Verification items for the finished model (mm, model axes). A direction names the side the tool comes from. Coordinates: 2 decimals unless noted, no trailing zeros. Loops run counter-clockwise (first coordinate to the right, second up) from the corner with the lowest first, then second, coordinate; pieces in that order, holes last. Notation, with made-up numbers: (85, 75.25) -> (111, 75.25) arc R22 cw to (111, 90.25) -> close; hole circle Ø7 at (33.5, 59). An arc over 180 degrees is marked (long way). Write item = value, one per line.
```python
from build123d import *

# Parameters (mm, degrees)
BOSS_EXTRUDE1_START     = 3.25
BOSS_EXTRUDE1_OUTLINE_W = 176
BOSS_EXTRUDE1_OUTLINE_H = 126
BOSS_EXTRUDE1_DEPTH     = 6
BOSS_EXTRUDE2_DEPTH     = 3.3
BOSS_EXTRUDE4_DEPTH     = 1
SKETCH7_W               = 12.05
SKETCH7_H               = 9
CUT_EXTRUDE1_DEPTH      = 6
BOSS_EXTRUDE5_DEPTH     = 3.3
BOSS_EXTRUDE7_DEPTH     = 1
BOSS_EXTRUDE8_START     = 2.6
BOSS_EXTRUDE8_DEPTH     = 2.6
BOSS_EXTRUDE9_START     = 0.7
BOSS_EXTRUDE9_DEPTH     = 0.7
BOSS_EXTRUDE10_START    = 1
BOSS_EXTRUDE10_DEPTH    = 1
SKETCH14_W              = 12.7
SKETCH14_H              = 3.5
SKETCH14_W_2            = 3.5
SKETCH14_H_2            = 25.4
CUT_EXTRUDE2_DEPTH      = 6.5116
CUT_EXTRUDE3_REACH      = 194.673
SKETCH15_R              = 4
CUT_EXTRUDE4_DEPTH      = 4.3
FILLET1_R               = 3
CUT_EXTRUDE5_START      = -4.8616
CUT_EXTRUDE5_DEPTH      = 4.8616
SKETCH19_W              = 176.2
SKETCH19_H              = 126.4
CUT_EXTRUDE6_DEPTH      = 3
SKETCH16_R              = 4
SKETCH16_R_2            = 2.1
BOSS_EXTRUDE11_DEPTH    = 4.25
SKETCH20_W              = 129.139207087
SKETCH20_H              = 3
SKETCH20_W_2            = 9.439207087
SKETCH20_W_3            = 158.5
BOSS_EXTRUDE12_DEPTH    = 4.25


# Read off the part's stored shape, not the designer's step: Boss-Extrude1, Cut-Extrude5
with BuildPart() as part:
    # Boss-Extrude1 outline → Boss-Extrude1 (new body)
    with BuildSketch(Plane.XY.offset(BOSS_EXTRUDE1_START)):
        with Locations((-88, 0)):
            Rectangle(BOSS_EXTRUDE1_OUTLINE_W, BOSS_EXTRUDE1_OUTLINE_H)
    extrude(amount=BOSS_EXTRUDE1_DEPTH)

    # Sketch3 → Boss-Extrude2 (add)
    with BuildSketch(Plane.ZY.offset(176)):
        with BuildLine():
            Line((9.25, -63), (9.25, 63))
            Line((9.25, 63), (-1.6116, 63))
            Line((-1.6116, 63), (-1.6116, 12.5))
            Line((-1.6116, 12.5), (0.4, 12.5))
            ThreePointArc((0.4, 12.5), (3.228427125, 11.328427125), (4.4, 8.5))
            Line((4.4, 8.5), (4.4, -8.5))
            ThreePointArc((4.4, -8.5), (3.228427125, -11.328427125), (0.4, -12.5))
            Line((0.4, -12.5), (-1.6116, -12.5))
            Line((-1.6116, -12.5), (-1.6116, -63))
            Line((-1.6116, -63), (9.25, -63))
        make_face()
    extrude(amount=BOSS_EXTRUDE2_DEPTH)

    # Sketch6 → Boss-Extrude4 (add)
    with BuildSketch(Plane.ZY.offset(179.3)):
        with BuildLine():
            Line((9.25, -63), (9.25, 63))
            Line((9.25, 63), (-1.6116, 63))
            Line((-1.6116, 63), (-1.6116, 11.25))
            Line((-1.6116, 11.25), (0.4, 11.25))
            ThreePointArc((0.4, 11.25), (2.415254326, 10.415254326), (3.25, 8.4))
            Line((3.25, 8.4), (3.25, -8.4))
            ThreePointArc((3.25, -8.4), (2.415254326, -10.415254326), (0.4, -11.25))
            Line((0.4, -11.25), (-1.6116, -11.25))
            Line((-1.6116, -11.25), (-1.6116, -63))
            Line((-1.6116, -63), (9.25, -63))
        make_face()
    extrude(amount=BOSS_EXTRUDE4_DEPTH)

    # Sketch7 → Cut-Extrude1 (cut)
    with BuildSketch(Plane(origin=(0, 0, 3.25), x_dir=(-1, 0, 0), z_dir=(0, 0, -1))):
        with Locations((138.325, -13.3)):
            Rectangle(SKETCH7_W, SKETCH7_H)
    extrude(amount=-CUT_EXTRUDE1_DEPTH, mode=Mode.SUBTRACT)

    # Sketch8 → Boss-Extrude5 (add)
    with BuildSketch(Plane.XZ.offset(63)):
        with BuildLine():
            Line((0, 9.25), (-180.3, 9.25))
            Line((-180.3, 9.25), (-180.3, -1.6116))
            Line((-180.3, -1.6116), (-11.957378406, -1.6116))
            ThreePointArc((-11.957378406, -1.6116), (-11.96744863, 2.394191566), (-8.5, 4.4))
            Line((-8.5, 4.4), (0, 4.4))
            Line((0, 4.4), (0, 9.25))
        make_face()
    extrude(amount=BOSS_EXTRUDE5_DEPTH)

    # Sketch10 → Boss-Extrude7 (add)
    with BuildSketch(Plane.XZ.offset(66.3)):
        with BuildLine():
            Line((0, 9.25), (-180.3, 9.25))
            Line((-180.3, 9.25), (-180.3, -1.6116))
            Line((-180.3, -1.6116), (-11.25, -1.6116))
            Line((-11.25, -1.6116), (-11.25, 0.4))
            ThreePointArc((-11.25, 0.4), (-10.415254326, 2.415254326), (-8.4, 3.25))
            Line((-8.4, 3.25), (0, 3.25))
            Line((0, 3.25), (0, 9.25))
        make_face()
    extrude(amount=BOSS_EXTRUDE7_DEPTH)

    # Sketch11 → Boss-Extrude8 (add)
    with BuildSketch(Plane(origin=(0, 63, 0), x_dir=(1, 0, 0), z_dir=(0, 1, 0)).offset(BOSS_EXTRUDE8_START)):
        with BuildLine():
            Line((-180.3, -9.25), (0, -9.25))
            Line((0, -9.25), (0, -4.4))
            Line((0, -4.4), (-8.5, -4.4))
            ThreePointArc((-8.5, -4.4), (-11.96744863, -2.394191566), (-11.957378406, 1.6116))
            Line((-11.957378406, 1.6116), (-180.3, 1.6116))
            Line((-180.3, 1.6116), (-180.3, -9.25))
        make_face()
    extrude(amount=-BOSS_EXTRUDE8_DEPTH)

    # Sketch12 → Boss-Extrude9 (add)
    with BuildSketch(Plane(origin=(0, 65.6, 0), x_dir=(1, 0, 0), z_dir=(0, 1, 0)).offset(BOSS_EXTRUDE9_START)):
        with BuildLine():
            Line((-180.3, -9.25), (0, -9.25))
            Line((0, -9.25), (0, -4.4))
            Line((0, -4.4), (-8.5, -4.4))
            ThreePointArc((-8.5, -4.4), (-11.96744863, -2.394191566), (-11.957378406, 1.6116))
            Line((-11.957378406, 1.6116), (-180.3, 1.6116))
            Line((-180.3, 1.6116), (-180.3, -9.25))
        make_face()
    extrude(amount=-BOSS_EXTRUDE9_DEPTH)

    # Sketch13 → Boss-Extrude10 (add)
    with BuildSketch(Plane(origin=(0, 66.3, 0), x_dir=(1, 0, 0), z_dir=(0, 1, 0)).offset(BOSS_EXTRUDE10_START)):
        with BuildLine():
            Line((-180.3, -9.25), (0, -9.25))
            Line((0, -9.25), (0, -3.25))
            Line((0, -3.25), (-8.4, -3.25))
            ThreePointArc((-8.4, -3.25), (-10.415254326, -2.415254326), (-11.25, -0.4))
            Line((-11.25, -0.4), (-11.25, 1.6116))
            Line((-11.25, 1.6116), (-180.3, 1.6116))
            Line((-180.3, 1.6116), (-180.3, -9.25))
        make_face()
    extrude(amount=-BOSS_EXTRUDE10_DEPTH)

    # Sketch14 → Cut-Extrude2 (cut)
    with BuildSketch(Plane(origin=(0, 0, -1.6116), x_dir=(-1, 0, 0), z_dir=(0, 0, -1))):
        with Locations((6.35, 64.75)):
            Rectangle(SKETCH14_W, SKETCH14_H)
        with Locations((177.75, 0)):
            Rectangle(SKETCH14_W_2, SKETCH14_H_2)
        with Locations((6.35, -64.75)):
            Rectangle(SKETCH14_W, SKETCH14_H)
    extrude(amount=-CUT_EXTRUDE2_DEPTH, mode=Mode.SUBTRACT)

    # Sketch15 → Cut-Extrude3 (cut, up to next)
    with BuildSketch(Plane.ZY.offset(180.3), mode=Mode.PRIVATE) as cut_extrude3_sk1:
        with Locations((-3.6116, -37.125)):
            Circle(SKETCH15_R)
    cut_extrude3_tool1 = extrude(cut_extrude3_sk1.sketch, amount=-CUT_EXTRUDE3_REACH, mode=Mode.PRIVATE) & part.part
    add(cut_extrude3_tool1.solids().sort_by_distance((-180.3, -37.125, -3.6116))[0], mode=Mode.SUBTRACT)

    # Sketch17 → Cut-Extrude4 (cut)
    with BuildSketch(Plane(origin=(0, 67.3, 0), x_dir=(1, 0, 0), z_dir=(0, 1, 0))):
        with BuildLine():
            Line((-28.4716, -5.0716), (-34.7284, -5.0716))
            ThreePointArc((-34.7284, -5.0716), (-38.07, -1.73), (-34.7284, 1.6116))
            Line((-34.7284, 1.6116), (-28.4716, 1.6116))
            ThreePointArc((-28.4716, 1.6116), (-25.13, -1.73), (-28.4716, -5.0716))
        make_face()
    extrude(amount=-CUT_EXTRUDE4_DEPTH, mode=Mode.SUBTRACT)

    # Fillet1
    fillet1_edges = [part.edges().sort_by_distance(p)[0] for p in [
        (-34.7284, 65.15, -1.6116),
    ]]
    fillet(fillet1_edges, radius=FILLET1_R)
    fillet1_2_edges = [part.edges().sort_by_distance(p)[0] for p in [
        (-28.4716, 65.15, -1.6116),
    ]]
    fillet(fillet1_2_edges, radius=FILLET1_R)

    # Cut-Extrude5 outline → Cut-Extrude5 (cut)
    with BuildSketch(Plane(origin=(0, 0, -1.6116), x_dir=(-1, 0, 0), z_dir=(0, 0, -1)).offset(CUT_EXTRUDE5_START)):
        Polygon((176, 63), (176, -63), (0, -63), (0, -63.2), (176.2, -63.2), (176.2, 63.2), (0, 63.2), (0, 63), align=None)
    extrude(amount=CUT_EXTRUDE5_DEPTH, mode=Mode.SUBTRACT)

    # Sketch19 → Cut-Extrude6 (cut)
    with BuildSketch(Plane(origin=(0, 0, 3.25), x_dir=(-1, 0, 0), z_dir=(0, 0, -1))):
        with Locations((88.1, 0)):
            Rectangle(SKETCH19_W, SKETCH19_H)
    extrude(amount=-CUT_EXTRUDE6_DEPTH, mode=Mode.SUBTRACT)

    # Sketch16 → Boss-Extrude11 (add)
    # profile 1 of 3: a face of its own
    with BuildSketch(Plane(origin=(0, 0, 6.25), x_dir=(-1, 0, 0), z_dir=(0, 0, -1))):
        with Locations(Location((156.5, 38, 0), (0, 0, 270))):
            Circle(SKETCH16_R)
        with Locations((156.5, 38)):
            Circle(SKETCH16_R_2, mode=Mode.SUBTRACT)
    # profile 2 of 3: a face of its own
    with BuildSketch(Plane(origin=(0, 0, 6.25), x_dir=(-1, 0, 0), z_dir=(0, 0, -1))):
        with Locations(Location((23.5, 38, 0), (0, 0, 270))):
            Circle(SKETCH16_R)
        with Locations((23.5, 38)):
            Circle(SKETCH16_R_2, mode=Mode.SUBTRACT)
    # profile 3 of 3: a face of its own
    with BuildSketch(Plane(origin=(0, 0, 6.25), x_dir=(-1, 0, 0), z_dir=(0, 0, -1))):
        with Locations(Location((123.5, -32, 0), (0, 0, 270))):
            Circle(SKETCH16_R)
        with Locations((123.5, -32)):
            Circle(SKETCH16_R_2, mode=Mode.SUBTRACT)
    extrude(amount=BOSS_EXTRUDE11_DEPTH)

    # Sketch20 → Boss-Extrude12 (add)
    with BuildSketch(Plane(origin=(0, 0, 6.25), x_dir=(-1, 0, 0), z_dir=(0, 0, -1))):
        with Locations((108.630396457, 61.7)):
            Rectangle(SKETCH20_W, SKETCH20_H)
        with Locations((17.419603544, 61.7)):
            Rectangle(SKETCH20_W_2, SKETCH20_H)
        Polygon((173.2, 17.7), (176.2, 17.7), (176.2, 63.2), (173.2, 63.2), (173.2, 60.2), align=None)
        with Locations((96.95, -61.7)):
            Rectangle(SKETCH20_W_3, SKETCH20_H)
    extrude(amount=BOSS_EXTRUDE12_DEPTH)


solid = part.part
```
1) Tool access check on faces 1 (the face through (-155, 36, 2)), 2 (the face through (-127.466, -31.479, 4.155)), 3 (the face through (0, 1, 8)). Record the directions out of +Z, -Z, +X, -X, +Y, -Y that give a thin tool (end or side, any length) a straight path to the whole face; none if there is none.
Ans:
face_1 = -Z, +X
face_2 = -Z
face_3 = +Z, -Z, +X, +Y, -Y
2) Depth check by flat-ended pin: pin 1 Ø1.7 at (x, y) = (-178.5, -4) entering from -Z; pin 2 Ø2.5 at (x, y) = (-124.5, -33) entering from -Z; pin 3 Ø4 at (y, z) = (-23.5, 0.5) entering from +X. Enter the tip coordinate at first touch or a pass-through.
Ans:
pin_1 = 4.9
pin_2 = 2
pin_3 = -176.2
3) Release check for a two-part mould opening along Y. For faces 4 (the face through (-91, 67.3, 4)), 5 (the face through (-8, 66.5, 4)), 6 (the face through (-17, 65, -1.612)), 7 (the face through (-91, -67.3, 4)) record: pulls with the +Y half, pulls with the -Y half, needs draft (parallel to the pull), parting line crosses it, or undercut.
Ans:
face_4 = pulls with the +Y half
face_5 = undercut
face_6 = needs draft
face_7 = pulls with the -Y half
4) Sectioned sample at B-B, the plane y = -49. Record the cut outline in (x, z), plus the area to 3 significant figures.
Ans:
outline = (-180.3, -1.61) -> (-176.2, -1.61) -> (-176.2, 6.25) -> (0, 6.25) -> (0, 9.25) -> (-180.3, 9.25) -> close
area = 573 mm2
5) Material ranges on line 1 (Y direction, x = -23.5, z = 5.15); line 2 (Y direction, x = -156.5, z = 3.05); line 3 (Y direction, x = -109.5, z = 2.75), recorded low to high.
Ans:
line_1 = -67.3 to -60.2, 34 to 35.9, 40.1 to 42, 63.2 to 67.3
line_2 = -67.3 to -60.2, 34 to 35.9, 40.1 to 42, 60.2 to 67.3
line_3 = -67.3 to -60.2, 60.2 to 67.3
6) Sectioned sample at C-C, the plane x = -73. Record the cut outline in (y, z).
Ans:
outline = (-67.3, -1.61) -> (-63.2, -1.61) -> (-63.2, 2) -> (-60.2, 2) -> (-60.2, 6.25) -> (60.2, 6.25) -> (60.2, 2) -> (63.2, 2) -> (63.2, -1.61) -> (67.3, -1.61) -> (67.3, 9.25) -> (-67.3, 9.25) -> close
7) Sectioned sample at A-A, the plane x = -156.5. Record the cut outline in (y, z).
Ans:
outline = (-67.3, -1.61) -> (-63.2, -1.61) -> (-63.2, 2) -> (-60.2, 2) -> (-60.2, 6.25) -> (34, 6.25) -> (34, 2) -> (35.9, 2) -> (35.9, 6.25) -> (40.1, 6.25) -> (40.1, 2) -> (42, 2) -> (42, 6.25) -> (60.2, 6.25) -> (60.2, 2) -> (63.2, 2) -> (63.2, -1.61) -> (67.3, -1.61) -> (67.3, 9.25) -> (-67.3, 9.25) -> close
